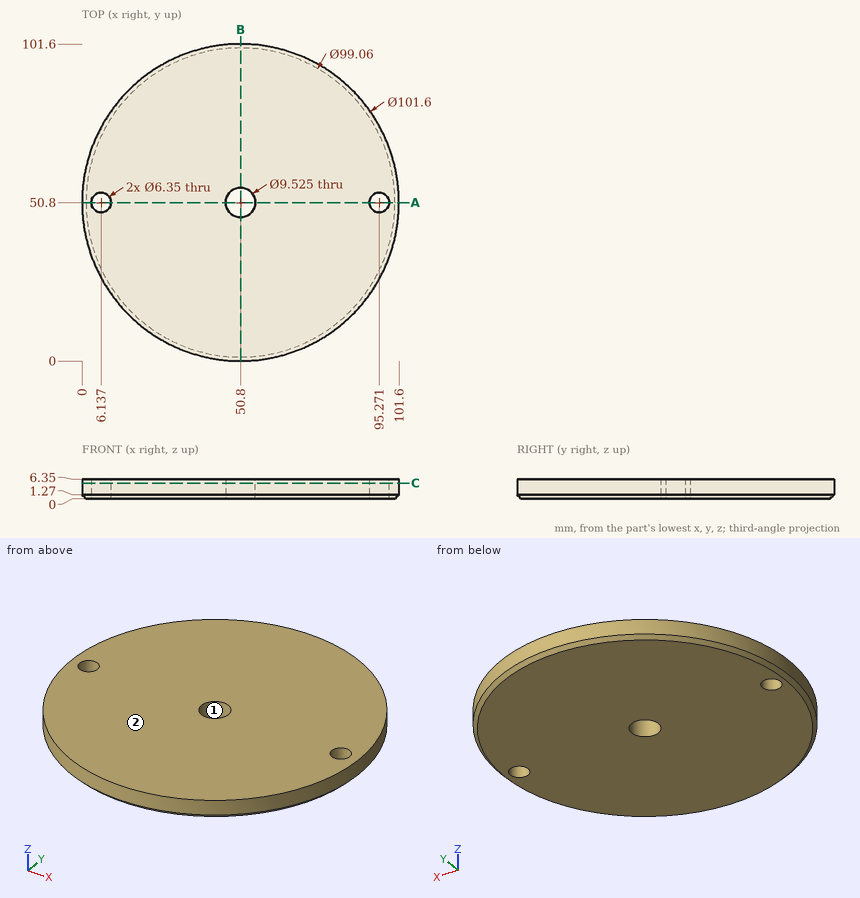
The drawing under review shows one solid part. Ordinate dimensions are in mm from its lowest x, y, z. Give positions to 0.01 mm unless a question says otherwise; leave off trailing zeros. Order: outer loops, then holes, each group sorted by start corner. A loop starts at its lowest first (then second) coordinate and runs counter-clockwise, first axis right, second up. Notation, with made-up numbers: (-21.75, 43.25) - (36.25, 43.25) arc R16 ccw to (36.25, 52.25) - close; hole circle Ø9 at (-34.5, 54.25). An arc over 180 degrees is marked (long way). Answer as a JSON object with one key per item and string values. Group by question number.
Item 1: Take a section at A-A on y = 50.8. Give the boundary of the cut face in (x, z).
Item 2: Clearance check with flat-ended pins moving along their axes: pin 1 Ø5 at (x, y) = (6.14, 50.8) entering from +Z; pin 2 Ø1 at (x, z) = (16, 1) entering from +Y; pin 3 Ø2 at (y, z) = (40.5, 3) entering from -X; pin 4 Ø1 at (y, z) = (47.5, 5.5) entering from -X. State where each tip first meets the part, or that it passes through.
Item 3: Wall thickness on line 1 along Y through (x, z) = (51, 6); line 2 along Y through (x, z) = (8, 4.75) (1 decimal); line 3 along X through (y, z) = (80, 1.5): over which ranges is each line inside the solid? List them lowest first.
Item 4: Draft analysis for pull direction Y (two halves, no side actions). For the marked faces 1 and 2, state which applies: pulls with the +Y half, pulls with the -Y half, needs draft (parallel to the pull), parting line crosses it, or undercut.
Item 5: Take a section at C-C on z = 5. Give the number of separate pieces and of enclosed holes in the cut face, and give its area (3 significant figures).
Item 6: Take a section at B-B on x = 50.8. Give the boundary of the cut face in (y, z).
Reported:
{
 "1": {"outline": "(0, 1.27) - (1.27, 0) - (2.96, 0) - (2.96, 6.35) - (0, 6.35) - close; (9.31, 0) - (46.04, 0) - (46.04, 6.35) - (9.31, 6.35) - close; (55.56, 0) - (92.1, 0) - (92.1, 6.35) - (55.56, 6.35) - close; (98.45, 0) - (100.33, 0) - (101.6, 1.27) - (101.6, 6.35) - (98.45, 6.35) - close"},
 "2": {"pin 1": "through", "pin 2": "y = 88.2", "pin 3": "x = 0.86", "pin 4": "x = 0.08"},
 "3": {"line 1": "0 to 46.04, 55.56 to 101.6", "line 2": "23.4 to 48.2, 53.4 to 78.2", "line 3": "9.23 to 92.37"},
 "4": {"face 1": "undercut", "face 2": "needs draft"},
 "5": {"separate pieces": "1", "enclosed holes": "3", "area": "7,970 mm^2"},
 "6": {"outline": "(0, 1.27) - (1.27, 0) - (46.04, 0) - (46.04, 6.35) - (0, 6.35) - close; (55.56, 0) - (100.33, 0) - (101.6, 1.27) - (101.6, 6.35) - (55.56, 6.35) - close"}
}
